Design review of the part built by this model. Coordinates are the model's own, in mm. A direction names the side the tool comes from. Coordinates: 2 decimals unless noted, no trailing zeros. Answer as a JSON object with one key per item and string values.
from build123d import *

# Parameters (mm, degrees)
F0_R          = 39
F0_R_2        = 2.325
F1_DEPTH      = 4
F2_R          = 3
F4_R          = 2.325
F5_DEPTH      = 3.5
F6_T4_DEPTH   = 7.9987755183
F6_T10_DEPTH  = 7.9987755183
F6_T16_DEPTH  = 7.9987755183
F6_T22_DEPTH  = 7.9987755183
F6_T28_DEPTH  = 7.9987755183
F6_T34_DEPTH  = 7.9987755183
F6_T38_ANGLE  = 270
F6_T40_ANGLE  = 90
F6_T42_ANGLE  = 90
F6_T44_ANGLE  = 270
F6_T49_DEPTH  = 7.9987755183
F6_T53_DEPTH  = 7.9987755183
F6_T60_DEPTH  = 7.9987755183
F6_T64_DEPTH  = 7.9987755183
F6_T71_DEPTH  = 7.9987755183
F6_T75_DEPTH  = 7.9987755183
F6_T82_DEPTH  = 7.9987755183
F6_T86_DEPTH  = 7.9987755183
F6_T93_DEPTH  = 7.9987755183
F6_T97_DEPTH  = 7.9987755183
F6_T104_DEPTH = 7.9987755183
F6_T108_DEPTH = 7.9987755183
F7_R          = 7.35
F8_DEPTH      = 25
F9_SIZE       = 2


# Not quite as in the source:
# - a fillet or chamfer that OpenCascade refuses, or shapes differently, is made with other operations: its cross-section is extruded or revolved along the edge and cut away or added


with BuildPart() as f1:
    # F0 (on Top) → F1 (new body, symmetric)
    with BuildSketch(Plane.XY):
        Circle(F0_R)
        Circle(F0_R_2, mode=Mode.SUBTRACT)
    extrude(amount=F1_DEPTH, both=True)

    # F2 (on Right) → F3 (revolve, cut)
    with BuildSketch(Plane.YZ):
        with Locations((-39, 0)):
            Circle(F2_R)
    revolve(axis=Axis((0, 0, 0), (0, 0, -1)), mode=Mode.SUBTRACT)

    # F4 (on face) → F5 (cut)
    with BuildSketch(Plane.XY.offset(4)):
        Polygon((-4.7, 2.7135462652), (-4.7, -2.7135462652), (0, -5.4270925304), (4.7, -2.7135462652), (4.7, 2.7135462652), (0, 5.4270925304), align=None)
        Circle(F4_R, mode=Mode.SUBTRACT)
    extrude(amount=-F5_DEPTH, mode=Mode.SUBTRACT)

    # F6: chamfer of 0.5 on 10 edges, made by hand


with BuildPart() as f6_tool2:
    # F6_s3 → F6_t4 (new body)
    with BuildSketch(Plane(origin=(3.463571399, -1.9996938796, 0), x_dir=(0, 0, 1), z_dir=(-0.8660254038, 0.5, 0))):
        Polygon((4, 5.2), (3.5, 4.7), (4, 4.7), align=None)
    extrude(amount=F6_T4_DEPTH)

    split(bisect_by=Plane.YZ.offset(4.7), keep=Keep.BOTTOM)

    split(bisect_by=Plane(origin=(-2.35, 4.0703193978, 0), x_dir=(0, 0, 1), z_dir=(0.5, -0.8660254038, 0)), keep=Keep.TOP)


with BuildPart() as f1_1:
    add(f1.part)

    # F6_t1: cut F6_tool2
    add(f6_tool2.part, mode=Mode.SUBTRACT)


with BuildPart() as f6_tool8:
    # F6_s9 → F6_t10 (new body)
    with BuildSketch(Plane.XZ.offset(3.9993877592)):
        Polygon((5.2, 4), (4.7, 3.5), (4.7, 4), align=None)
    extrude(amount=-F6_T10_DEPTH)

    split(bisect_by=Plane(origin=(2.35, -4.0703193978, 0), x_dir=(0, 0, 1), z_dir=(-0.5, 0.8660254038, 0)), keep=Keep.TOP)

    split(bisect_by=Plane(origin=(2.35, 4.0703193978, 0), x_dir=(0, 0, 1), z_dir=(-0.5, -0.8660254038, 0)), keep=Keep.TOP)


with BuildPart() as f1_2:
    add(f1_1.part)

    # F6_t7: cut F6_tool8
    add(f6_tool8.part, mode=Mode.SUBTRACT)


with BuildPart() as f6_tool14:
    # F6_s15 → F6_t16 (new body)
    with BuildSketch(Plane(origin=(-3.463571399, -1.9996938796, 0), x_dir=(0, 0, 1), z_dir=(0.8660254038, 0.5, 0))):
        Polygon((4, 5.2), (3.5, 4.7), (4, 4.7), align=None)
    extrude(amount=F6_T16_DEPTH)

    split(bisect_by=Plane(origin=(-2.35, -4.0703193978, 0), x_dir=(0, 0, 1), z_dir=(0.5, 0.8660254038, 0)), keep=Keep.TOP)

    split(bisect_by=Plane.YZ.offset(4.7), keep=Keep.BOTTOM)


with BuildPart() as f1_3:
    add(f1_2.part)

    # F6_t13: cut F6_tool14
    add(f6_tool14.part, mode=Mode.SUBTRACT)


with BuildPart() as f6_tool20:
    # F6_s21 → F6_t22 (new body)
    with BuildSketch(Plane(origin=(-3.463571399, 1.9996938796, 0), x_dir=(0, 0, 1), z_dir=(0.8660254038, -0.5, 0))):
        Polygon((4, 5.2), (3.5, 4.7), (4, 4.7), align=None)
    extrude(amount=F6_T22_DEPTH)

    split(bisect_by=Plane.YZ.offset(-4.7), keep=Keep.TOP)

    split(bisect_by=Plane(origin=(2.35, -4.0703193978, 0), x_dir=(0, 0, 1), z_dir=(-0.5, 0.8660254038, 0)), keep=Keep.TOP)


with BuildPart() as f1_4:
    add(f1_3.part)

    # F6_t19: cut F6_tool20
    add(f6_tool20.part, mode=Mode.SUBTRACT)


with BuildPart() as f6_tool26:
    # F6_s27 → F6_t28 (new body)
    with BuildSketch(Plane.XZ.offset(-3.9993877592)):
        Polygon((-5.2, 4), (-4.7, 3.5), (-4.7, 4), align=None)
    extrude(amount=F6_T28_DEPTH)

    split(bisect_by=Plane(origin=(-2.35, -4.0703193978, 0), x_dir=(0, 0, 1), z_dir=(0.5, 0.8660254038, 0)), keep=Keep.TOP)

    split(bisect_by=Plane(origin=(-2.35, 4.0703193978, 0), x_dir=(0, 0, 1), z_dir=(0.5, -0.8660254038, 0)), keep=Keep.TOP)


with BuildPart() as f1_5:
    add(f1_4.part)

    # F6_t25: cut F6_tool26
    add(f6_tool26.part, mode=Mode.SUBTRACT)


with BuildPart() as f6_tool32:
    # F6_s33 → F6_t34 (new body)
    with BuildSketch(Plane(origin=(3.463571399, 1.9996938796, 0), x_dir=(0, 0, 1), z_dir=(-0.8660254038, -0.5, 0))):
        Polygon((4, 5.2), (3.5, 4.7), (4, 4.7), align=None)
    extrude(amount=F6_T34_DEPTH)

    split(bisect_by=Plane.YZ.offset(-4.7), keep=Keep.TOP)

    split(bisect_by=Plane(origin=(2.35, 4.0703193978, 0), x_dir=(0, 0, 1), z_dir=(-0.5, -0.8660254038, 0)), keep=Keep.TOP)


with BuildPart() as f1_6:
    add(f1_5.part)

    # F6_t31: cut F6_tool32
    add(f6_tool32.part, mode=Mode.SUBTRACT)

    # F6_s37 → F6_t38 (revolve, cut)
    with BuildSketch(Plane.YZ):
        with BuildLine():
            Line((-39, -3.4641016151), (-38.5714285714, -2.9692299558))
            ThreePointArc((-38.5714285714, -2.9692299558), (-38.7780755038, -2.9917803258), (-39, -3))
            Line((-39, -3), (-39, -3.4641016151))
        make_face()
    revolve(axis=Axis((0, 0, -3), (0, 0, -1)), revolution_arc=F6_T38_ANGLE, mode=Mode.SUBTRACT)

    # F6_s39 → F6_t40 (revolve, cut)
    with BuildSketch(Plane.XZ):
        with BuildLine():
            Line((39, -3.4641016151), (38.5714285714, -2.9692299558))
            ThreePointArc((38.5714285714, -2.9692299558), (38.7780755038, -2.9917803258), (39, -3))
            Line((39, -3), (39, -3.4641016151))
        make_face()
    revolve(axis=Axis((0, 0, -3), (0, 0, -1)), revolution_arc=F6_T40_ANGLE, mode=Mode.SUBTRACT)

    # F6_s41 → F6_t42 (revolve, cut)
    with BuildSketch(Plane.XZ):
        with BuildLine():
            Line((38.5714285714, 2.9692299558), (39, 3.4641016151))
            Line((39, 3.4641016151), (39, 3))
            ThreePointArc((39, 3), (38.7780755038, 2.9917803258), (38.5714285714, 2.9692299558))
        make_face()
    revolve(axis=Axis((0, 0, 3), (0, 0, -1)), revolution_arc=F6_T42_ANGLE, mode=Mode.SUBTRACT)

    # F6_s43 → F6_t44 (revolve, cut)
    with BuildSketch(Plane.YZ):
        with BuildLine():
            Line((-38.5714285714, 2.9692299558), (-39, 3.4641016151))
            Line((-39, 3.4641016151), (-39, 3))
            ThreePointArc((-39, 3), (-38.7780755038, 2.9917803258), (-38.5714285714, 2.9692299558))
        make_face()
    revolve(axis=Axis((0, 0, 3), (0, 0, -1)), revolution_arc=F6_T44_ANGLE, mode=Mode.SUBTRACT)


with BuildPart() as f6_tool47:
    # F6_s48 → F6_t49 (new body)
    with BuildSketch(Plane.XZ.offset(3.9993877592)):
        Polygon((5.2, 4), (4.7, 3.5), (4.7, 4), align=None)
    extrude(amount=-F6_T49_DEPTH)

    split(bisect_by=Plane(origin=(2.35, 4.0703193978, 0), x_dir=(0, 0, 1), z_dir=(0.5, 0.8660254038, 0)), keep=Keep.TOP)


with BuildPart() as f6_tool51:
    # F6_s52 → F6_t53 (new body)
    with BuildSketch(Plane(origin=(3.463571399, -1.9996938796, 0), x_dir=(0, 0, 1), z_dir=(-0.8660254038, 0.5, 0))):
        Polygon((4, 5.2), (3.5, 4.7), (4, 4.7), align=None)
    extrude(amount=F6_T53_DEPTH)

    split(bisect_by=Plane.YZ.offset(4.7), keep=Keep.TOP)


with BuildPart() as f6_tool47_1:
    add(f6_tool47.part)

    # F6_t55: intersect F6_tool51
    add(f6_tool51.part, mode=Mode.INTERSECT)


with BuildPart() as f1_7:
    add(f1_6.part)

    # F6_t45: cut F6_tool47
    add(f6_tool47_1.part, mode=Mode.SUBTRACT)


with BuildPart() as f6_tool58:
    # F6_s59 → F6_t60 (new body)
    with BuildSketch(Plane(origin=(3.463571399, -1.9996938796, 0), x_dir=(0, 0, 1), z_dir=(-0.8660254038, 0.5, 0))):
        Polygon((4, 5.2), (3.5, 4.7), (4, 4.7), align=None)
    extrude(amount=F6_T60_DEPTH)

    split(bisect_by=Plane(origin=(-2.35, 4.0703193978, 0), x_dir=(0, 0, 1), z_dir=(-0.5, 0.8660254038, 0)), keep=Keep.TOP)


with BuildPart() as f6_tool62:
    # F6_s63 → F6_t64 (new body)
    with BuildSketch(Plane(origin=(3.463571399, 1.9996938796, 0), x_dir=(0, 0, 1), z_dir=(-0.8660254038, -0.5, 0))):
        Polygon((4, 5.2), (3.5, 4.7), (4, 4.7), align=None)
    extrude(amount=F6_T64_DEPTH)

    split(bisect_by=Plane(origin=(2.35, 4.0703193978, 0), x_dir=(0, 0, 1), z_dir=(0.5, 0.8660254038, 0)), keep=Keep.TOP)


with BuildPart() as f6_tool58_1:
    add(f6_tool58.part)

    # F6_t66: intersect F6_tool62
    add(f6_tool62.part, mode=Mode.INTERSECT)


with BuildPart() as f1_8:
    add(f1_7.part)

    # F6_t56: cut F6_tool58
    add(f6_tool58_1.part, mode=Mode.SUBTRACT)


with BuildPart() as f6_tool69:
    # F6_s70 → F6_t71 (new body)
    with BuildSketch(Plane(origin=(-3.463571399, -1.9996938796, 0), x_dir=(0, 0, 1), z_dir=(0.8660254038, 0.5, 0))):
        Polygon((4, 5.2), (3.5, 4.7), (4, 4.7), align=None)
    extrude(amount=F6_T71_DEPTH)

    split(bisect_by=Plane.YZ.offset(4.7), keep=Keep.TOP)


with BuildPart() as f6_tool73:
    # F6_s74 → F6_t75 (new body)
    with BuildSketch(Plane.XZ.offset(3.9993877592)):
        Polygon((5.2, 4), (4.7, 3.5), (4.7, 4), align=None)
    extrude(amount=-F6_T75_DEPTH)

    split(bisect_by=Plane(origin=(2.35, -4.0703193978, 0), x_dir=(0, 0, 1), z_dir=(0.5, -0.8660254038, 0)), keep=Keep.TOP)


with BuildPart() as f6_tool69_1:
    add(f6_tool69.part)

    # F6_t77: intersect F6_tool73
    add(f6_tool73.part, mode=Mode.INTERSECT)


with BuildPart() as f1_9:
    add(f1_8.part)

    # F6_t67: cut F6_tool69
    add(f6_tool69_1.part, mode=Mode.SUBTRACT)


with BuildPart() as f6_tool80:
    # F6_s81 → F6_t82 (new body)
    with BuildSketch(Plane(origin=(-3.463571399, 1.9996938796, 0), x_dir=(0, 0, 1), z_dir=(0.8660254038, -0.5, 0))):
        Polygon((4, 5.2), (3.5, 4.7), (4, 4.7), align=None)
    extrude(amount=F6_T82_DEPTH)

    split(bisect_by=Plane(origin=(2.35, -4.0703193978, 0), x_dir=(0, 0, 1), z_dir=(0.5, -0.8660254038, 0)), keep=Keep.TOP)


with BuildPart() as f6_tool84:
    # F6_s85 → F6_t86 (new body)
    with BuildSketch(Plane(origin=(-3.463571399, -1.9996938796, 0), x_dir=(0, 0, 1), z_dir=(0.8660254038, 0.5, 0))):
        Polygon((4, 5.2), (3.5, 4.7), (4, 4.7), align=None)
    extrude(amount=F6_T86_DEPTH)

    split(bisect_by=Plane(origin=(-2.35, -4.0703193978, 0), x_dir=(0, 0, 1), z_dir=(-0.5, -0.8660254038, 0)), keep=Keep.TOP)


with BuildPart() as f6_tool80_1:
    add(f6_tool80.part)

    # F6_t88: intersect F6_tool84
    add(f6_tool84.part, mode=Mode.INTERSECT)


with BuildPart() as f1_10:
    add(f1_9.part)

    # F6_t78: cut F6_tool80
    add(f6_tool80_1.part, mode=Mode.SUBTRACT)


with BuildPart() as f6_tool91:
    # F6_s92 → F6_t93 (new body)
    with BuildSketch(Plane.XZ.offset(-3.9993877592)):
        Polygon((-5.2, 4), (-4.7, 3.5), (-4.7, 4), align=None)
    extrude(amount=F6_T93_DEPTH)

    split(bisect_by=Plane(origin=(-2.35, -4.0703193978, 0), x_dir=(0, 0, 1), z_dir=(-0.5, -0.8660254038, 0)), keep=Keep.TOP)


with BuildPart() as f6_tool95:
    # F6_s96 → F6_t97 (new body)
    with BuildSketch(Plane(origin=(-3.463571399, 1.9996938796, 0), x_dir=(0, 0, 1), z_dir=(0.8660254038, -0.5, 0))):
        Polygon((4, 5.2), (3.5, 4.7), (4, 4.7), align=None)
    extrude(amount=F6_T97_DEPTH)

    split(bisect_by=Plane.YZ.offset(-4.7), keep=Keep.BOTTOM)


with BuildPart() as f6_tool91_1:
    add(f6_tool91.part)

    # F6_t99: intersect F6_tool95
    add(f6_tool95.part, mode=Mode.INTERSECT)


with BuildPart() as f1_11:
    add(f1_10.part)

    # F6_t89: cut F6_tool91
    add(f6_tool91_1.part, mode=Mode.SUBTRACT)


with BuildPart() as f6_tool102:
    # F6_s103 → F6_t104 (new body)
    with BuildSketch(Plane.XZ.offset(-3.9993877592)):
        Polygon((-5.2, 4), (-4.7, 3.5), (-4.7, 4), align=None)
    extrude(amount=F6_T104_DEPTH)

    split(bisect_by=Plane(origin=(-2.35, 4.0703193978, 0), x_dir=(0, 0, 1), z_dir=(-0.5, 0.8660254038, 0)), keep=Keep.TOP)


with BuildPart() as f6_tool106:
    # F6_s107 → F6_t108 (new body)
    with BuildSketch(Plane(origin=(3.463571399, 1.9996938796, 0), x_dir=(0, 0, 1), z_dir=(-0.8660254038, -0.5, 0))):
        Polygon((4, 5.2), (3.5, 4.7), (4, 4.7), align=None)
    extrude(amount=F6_T108_DEPTH)

    split(bisect_by=Plane.YZ.offset(-4.7), keep=Keep.BOTTOM)


with BuildPart() as f6_tool102_1:
    add(f6_tool102.part)

    # F6_t110: intersect F6_tool106
    add(f6_tool106.part, mode=Mode.INTERSECT)


with BuildPart() as f1_12:
    add(f1_11.part)

    # F6_t100: cut F6_tool102
    add(f6_tool102_1.part, mode=Mode.SUBTRACT)

    # F7 (on face) → F8 (cut)
    with BuildSketch(Plane.XY.offset(4)):
        with Locations((20, 0)):
            Circle(F7_R)
        with Locations((10, -17.3205080757)):
            Circle(F7_R)
        with Locations((-10, -17.3205080757)):
            Circle(F7_R)
        with Locations((-20, 0)):
            Circle(F7_R)
        with Locations((-10, 17.3205080757)):
            Circle(F7_R)
        with Locations((10, 17.3205080757)):
            Circle(F7_R)
    extrude(amount=-F8_DEPTH, mode=Mode.SUBTRACT)

    # F9
    f9_edges = [f1_12.edges().sort_by_distance(p)[0] for p in [
        (12.65, 0, 4),
        (2.65, -17.320508, 4),
        (-17.35, -17.320508, 4),
        (-27.35, 0, 4),
        (-17.35, 17.320508, 4),
        (2.65, 17.320508, 4),
        (-27.35, 0, -4),
        (-17.35, -17.320508, -4),
        (2.65, -17.320508, -4),
        (12.65, 0, -4),
        (2.65, 17.320508, -4),
        (-17.35, 17.320508, -4),
    ]]
    chamfer(f9_edges, length=F9_SIZE)


solid = f1_12.part
1) Add section A-A (y = -20). Count the separate pieces of the cut face and the enclosed holes in it, and give its area (3 significant figures).
Taken from the geometry:
{"separate pieces": "3", "enclosed holes": "0", "area": "266 mm2"}
2) Tool access review of faces 1 (the cylindrical face through (1.25, 1.96, -1.78)), 2 (the flat face through (2.383, 4.051, 2.021)): name each direction out of +Z, -Z, +X, -X, +Y, -Y from which nothing blocks a thin tool from reaching the whole face with its end or side.
Taken from the geometry:
{"face 1": "+Z, -Z", "face 2": "+Z"}
3) To check wall thickness, follow L1, parallel to X at y = -19, z = 0.25; L2, parallel to Y at x = 10, z = 1; L3, parallel to X at y = 5, z = -0.75. State the ranges of each line that lie inside material, in increasing order.
Taken from the geometry:
{"L1": "x = -30.59 to -17.16, -2.84 to 2.84, 17.16 to 30.59", "L2": "y = -34.76 to -24.67, -9.97 to 9.97, 24.67 to 34.76", "L3": "x = -35.75 to -25.39, -14.61 to 14.61, 25.39 to 35.75"}
4) Mouldability with a two-part tool opening along Y and no side actions: class faces 3 (the cylindrical face through (-5.077, 38.668, 3.736)), 4 (the cylindrical face through (-6.05, 23.52, 0.03)) as released by +Y, released by -Y, zero draft, split by the parting line, or undercut.
Taken from the geometry:
{"face 3": "split by the parting line", "face 4": "undercut"}
5) Insertion check: pin 1 Ø17 at (x, y) = (10, -17.32) entering from -Z; pin 2 Ø4.5 at (x, y) = (0.5, -1) entering from +Z; pin 3 Ø2 at (y, z) = (-10, -1) entering from +X. Each pin has a flat end and moves straight along its axis. Give the tip position at first contact, or say it passes through.
Taken from the geometry:
{"pin 1": "stops at z = -3.15", "pin 2": "stops at z = 0.5", "pin 3": "stops at x = 35.42"}
